Work out the finished part from the listing and answer in its coordinate system (mm). Face numbers are marked on the shaded views. A direction names the side the tool comes from. Coordinates: 2 decimals unless noted, no trailing zeros. Order: outer loops, then holes, each group sorted by start corner. A loop starts at its lowest first (then second) coordinate and runs counter-clockwise, first axis right, second up. Notation, with made-up numbers: M -19,34 L 37,34 A30 cw 37,59 Z; hole C 56.25,68.25 d5. An arc over 180 degrees is marked long. Use a Markdown table: item, result.
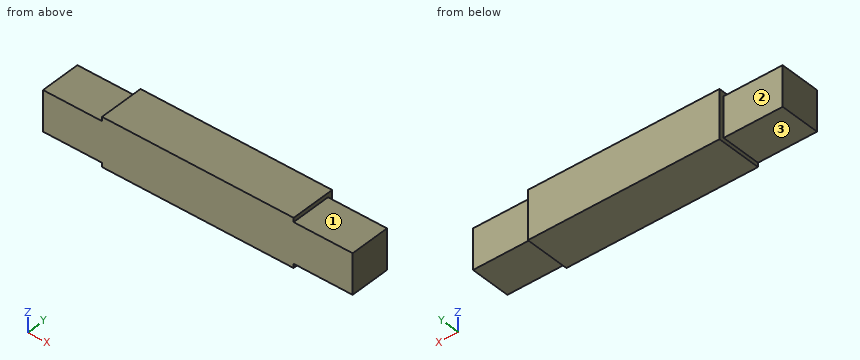
from build123d import *

# Parameters (mm, degrees)
SKETCH2_W             = 10.795
SKETCH2_H             = 7.366
BOSS_EXTRUDE1_DEPTH   = 7.366
BOSS_EXTRUDE1_2_DEPTH = 7.366
SKETCH2_4_W           = 35.052
SKETCH2_4_H           = 0.762
SKETCH2_4_H_2         = 7.366
BOSS_EXTRUDE2_DEPTH   = 8.255


with BuildPart() as part:
    # Sketch2 → Boss-Extrude1 (new body)
    with BuildSketch(Plane(origin=(0, 0, 0), x_dir=(1, 0, 0), z_dir=(0, 1, 0))):
        with Locations((-22.9235, 0)):
            Rectangle(SKETCH2_W, SKETCH2_H)
    extrude(amount=BOSS_EXTRUDE1_DEPTH)



with BuildPart() as body_2:
    # Sketch2 → Boss-Extrude1 2 (new body)
    with BuildSketch(Plane(origin=(0, 0, 0), x_dir=(1, 0, 0), z_dir=(0, 1, 0))):
        with Locations((22.9235, 0)):
            Rectangle(SKETCH2_W, SKETCH2_H)
    extrude(amount=BOSS_EXTRUDE1_2_DEPTH)


with BuildPart() as part_1:
    add(part.part)

    add(body_2.part)  # Boss-Extrude2 merges body 2
    # Sketch2_4 → Boss-Extrude2 (add)
    with BuildSketch(Plane(origin=(0, 0, 0), x_dir=(1, 0, 0), z_dir=(0, 1, 0))):
        with Locations((0, 4.064)):
            Rectangle(SKETCH2_4_W, SKETCH2_4_H)
        Rectangle(SKETCH2_4_W, SKETCH2_4_H_2)
        with Locations((0, -4.064)):
            Rectangle(SKETCH2_4_W, SKETCH2_4_H)
    extrude(amount=BOSS_EXTRUDE2_DEPTH)


solid = part_1.part
(1) A cutting plane is placed at B-B (y = 4). Determine the outline of the cut face in (x, z) (3 decimals), then the cut area to 3 significant figures.
Conclusion:
| item | result |
|---|---|
| outline | M -28.321,-3.683 L -17.526,-3.683 L -17.526,-4.445 L 17.526,-4.445 L 17.526,-3.683 L 28.321,-3.683 L 28.321,3.683 L 17.526,3.683 L 17.526,4.445 L -17.526,4.445 L -17.526,3.683 L -28.321,3.683 Z |
| area | 471 mm2 |
(2) Which of the six approach directions +Z, -Z, +X, -X, +Y, -Y give full straight-line access (tool end or side, diameter ignored) to the marked faces 1, 2 and 3?
Conclusion:
| item | result |
|---|---|
| face 1 | +Z, +X, +Y, -Y |
| face 2 | +Z, -Z, -X, +Y |
| face 3 | -Z, -X, +Y, -Y |
(3) A cutting plane is placed at A-A (z = 0). Determine the outline of the cut face in (x, y) (3 decimals), then the cut area to 3 significant figures.
Conclusion:
| item | result |
|---|---|
| outline | M -28.321,0 L 28.321,0 L 28.321,7.366 L 17.526,7.366 L 17.526,8.255 L -17.526,8.255 L -17.526,7.366 L -28.321,7.366 Z |
| area | 448 mm2 |
(4) A cutting plane is placed at C-C (x = -25). Determine the outline of the cut face in (y, z), then the cut area to 3 significant figures.
Conclusion:
| item | result |
|---|---|
| outline | M 0,-3.68 L 7.37,-3.68 L 7.37,3.68 L 0,3.68 Z |
| area | 54.3 mm2 |
(5) Straight lines are drawn through the part: L1, parallel to Z at x = 22.5, y = 2.25; L2, parallel to Y at x = 24, z = 2.5; L3, parallel to X at y = 8, z = -1.75. For each, find the intervals that lie inside material, in ascending order.
Conclusion:
| item | result |
|---|---|
| L1 | -3.68 to 3.68 |
| L2 | 0 to 7.37 |
| L3 | -17.53 to 17.53 |
(6) Given P1, Ø3.5, axis at x = -21, y = 5.5, coming from the -Z side; P2, Ø4, axis at x = 7.5, z = 2, coming from the -Y side; P3, Ø3.5, axis at x = 20.5, y = 2, coming from the +Z side, each flat-ended and moving along its own axis, determine where each tip first touches the part or whether it passes through.
Conclusion:
| item | result |
|---|---|
| P1 | z = -3.68 |
| P2 | y = 0 |
| P3 | z = 3.68 |
